```python
from build123d import *

# Parameters (mm, degrees)
BOSS_EXTRUDE2_DEPTH  = 10.2
SKETCH3_W            = 19.6
SKETCH3_H            = 4.3
BOSS_EXTRUDE3_DEPTH  = 2
FILLET3_R            = 1
SKETCH4_W            = 1.5
SKETCH4_H            = 7
BOSS_EXTRUDE4_DEPTH  = 20
SKETCH5_W            = 1.5
SKETCH5_H            = 7
BOSS_EXTRUDE5_DEPTH  = 20
SKETCH6_W            = 1.5
SKETCH6_H            = 6
BOSS_EXTRUDE7_DEPTH  = 3
SKETCH8_W            = 1.5
SKETCH8_H            = 6
BOSS_EXTRUDE8_DEPTH  = 16
FILLET4_R            = 1
FILLET5_R            = 1
BOSS_EXTRUDE10_DEPTH = 4
SKETCH12_R           = 2.4
CUT_EXTRUDE1_DEPTH   = 19


with BuildPart() as part:
    # Sketch1 → Boss-Extrude2 (new body)
    with BuildSketch(Plane(origin=(0, 0, 0), x_dir=(1, 0, 0), z_dir=(0, 1, 0))):
        with BuildLine():
            Line((-24.9, 16), (24.9, 16))
            ThreePointArc((24.9, 16), (26.879898987, 15.179898987), (27.7, 13.2))
            Line((27.7, 13.2), (27.7, -13.2))
            ThreePointArc((27.7, -13.2), (26.879898987, -15.179898987), (24.9, -16))
            Line((24.9, -16), (-24.9, -16))
            ThreePointArc((-24.9, -16), (-26.879898987, -15.179898987), (-27.7, -13.2))
            Line((-27.7, -13.2), (-27.7, 13.2))
            ThreePointArc((-27.7, 13.2), (-26.879898987, 15.179898987), (-24.9, 16))
        make_face()
    extrude(amount=BOSS_EXTRUDE2_DEPTH)

    # Sketch3 → Boss-Extrude3 (add)
    with BuildSketch(Plane(origin=(0, 0, -16), x_dir=(-1, 0, 0), z_dir=(0, 0, -1))):
        with Locations((-15.1, 5.1)):
            Rectangle(SKETCH3_W, SKETCH3_H)
    extrude(amount=BOSS_EXTRUDE3_DEPTH)

    # Fillet3
    fillet3_edges = [part.edges().sort_by_distance(p)[0] for p in [
        (5.3, 5.1, -18),
    ]]
    fillet(fillet3_edges, radius=FILLET3_R)

    # Sketch4 → Boss-Extrude4 (add)
    with BuildSketch(Plane.ZY.offset(27.7)):
        with Locations((-10.4, 5.1)):
            Rectangle(SKETCH4_W, SKETCH4_H)
    extrude(amount=BOSS_EXTRUDE4_DEPTH)

    # Sketch5 → Boss-Extrude5 (add)
    with BuildSketch(Plane.ZY.offset(27.7)):
        with Locations((10.4, 5.1)):
            Rectangle(SKETCH5_W, SKETCH5_H)
    extrude(amount=BOSS_EXTRUDE5_DEPTH)

    # Sketch6 → Boss-Extrude7 (add)
    with BuildSketch(Plane.XY.offset(16)):
        with Locations((-7.247043242, 5.066819201)):
            Rectangle(SKETCH6_W, SKETCH6_H)
    extrude(amount=BOSS_EXTRUDE7_DEPTH)

    # Sketch8 → Boss-Extrude8 (add)
    with BuildSketch(Plane.ZY.offset(7.997043242)):
        with Locations((18.25, 5.066819201)):
            Rectangle(SKETCH8_W, SKETCH8_H)
    extrude(amount=BOSS_EXTRUDE8_DEPTH)

    # Fillet4
    fillet4_edges = [part.edges().sort_by_distance(p)[0] for p in [
        (-7.997043242, 5.066819201, 17.5),
    ]]
    fillet(fillet4_edges, radius=FILLET4_R)

    # Fillet5
    fillet5_edges = [part.edges().sort_by_distance(p)[0] for p in [
        (-6.497043242, 5.066819201, 19),
    ]]
    fillet(fillet5_edges, radius=FILLET5_R)

    # Sketch11 → Boss-Extrude10 (add)
    with BuildSketch(Plane.XZ.offset(-2.95)):
        with BuildLine():
            Line((16.614530509, -19.138227367), (16.614530509, -16))
            Line((16.614530509, -16), (13.585469491, -16))
            Line((13.585469491, -16), (13.585469491, -19.138227367))
            ThreePointArc((13.585469491, -19.138227367), (15.1, -23.4), (16.614530509, -19.138227367))
        make_face()
    extrude(amount=-BOSS_EXTRUDE10_DEPTH)

    # Sketch12 → Cut-Extrude1 (cut)
    with BuildSketch(Plane(origin=(0, 10.2, 0), x_dir=(1, 0, 0), z_dir=(0, 1, 0))):
        with Locations(Location((0, 13.2, 0), (0, 0, 270))):
            Circle(SKETCH12_R)
    extrude(amount=-CUT_EXTRUDE1_DEPTH, mode=Mode.SUBTRACT)


solid = part.part
```
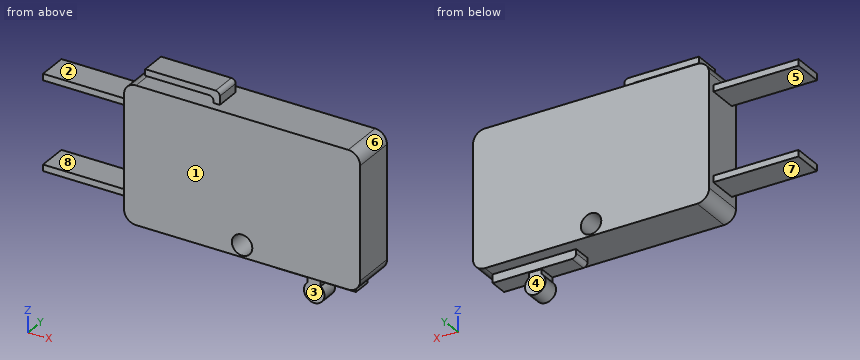
Could you check a few things on this model? Use its own coordinates, in mm. Face numbers are marked on the shaded views. A direction names the side the tool comes from. Round coordinates to 2 decimals unless told otherwise and drop trailing zeros. Loops run counter-clockwise (first coordinate to the right, second up) from the corner with the lowest first, then second, coordinate; pieces in that order, holes last.
Q1. I want a section at C-C (x = 15.1). Write out the boundary of the cut face in (y, z).
Q2. I want a section at D-D (x = 0). Write out the boundary of the cut face in (y, z), and give its area (3 significant figures).
Q3. On a 3-axis mill with a long thin cutter (end or side, diameter ignored), from which of +Z, -Z, +X, -X, +Y, -Y can I reach the whole of each face in a straight line? I mean the marked faces 1, 2, 3, 4 and 5. Say none if no direction works.
Q4. Thinking about a two-plate mould opening in Z: for the marked faces 6, 7 and 8, which applies, pulls with the +Z half, pulls with the -Z half, needs draft (parallel to the pull), parting line crosses it, or undercut?
Q5. Please list where these lines run through material, in increasing order: L1, parallel to Z at x = -32, y = 8; L2, parallel to Z at x = -16.5, y = 7.75; L3, parallel to X at y = 8.25, z = -13.2.
Q6. For P1, Ø1.5, axis at x = -36.5, z = -8, coming from the +Y side; P2, Ø5, axis at x = -31.5, z = 12.5, coming from the +Y side; P3, Ø5, axis at x = 5.5, y = 6, coming from the -Z side; P4, Ø2, axis at y = 4.5, z = -1, coming from the -X side, each with a flat end and sliding along its axis, tell me the tip position at first contact or that it passes through.
Q7. I want a section at A-A (x = -31). Write out the boundary of the cut face in (y, z), and give its area (3 significant figures).
Answer below:
1. outline: (0, -16) - (2.95, -16) - (2.95, -23.4) - (6.95, -23.4) - (6.95, -18) - (7.25, -18) - (7.25, -16) - (10.2, -16) - (10.2, 16) - (0, 16) - close
2. outline: (0, -16) - (10.2, -16) - (10.2, -15.6) - (0, -15.6) - close; (0, -10.8) - (10.2, -10.8) - (10.2, 16) - (0, 16) - close
2. area: 277 mm2
3. face 1: +Z, -Z, +X, -X, -Y
3. face 2: +Z, -X, +Y, -Y
3. face 3: -Z, +X, -X, -Y
3. face 4: -Z, +X, -X, +Y
3. face 5: -X, +Y, -Y
4. face 6: pulls with the +Z half
4. face 7: pulls with the -Z half
4. face 8: undercut
5. L1: z = -11.15 to -9.65, 9.65 to 11.15
5. L2: z = -16 to 16, 17.5 to 19
5. L3: x = -27.7 to -2.4, 2.4 to 27.7
6. P1: passes through
6. P2: stops at y = 8.6
6. P3: stops at z = -18
6. P4: stops at x = -27.7
7. outline: (1.6, -11.15) - (8.6, -11.15) - (8.6, -9.65) - (1.6, -9.65) - close; (1.6, 9.65) - (8.6, 9.65) - (8.6, 11.15) - (1.6, 11.15) - close
7. area: 21.0 mm2
